The drawing under review shows one solid part. Ordinate dimensions are in mm from its lowest x, y, z. A direction names the side the tool comes from. Give positions to 0.01 mm unless a question says otherwise; leave off trailing zeros. Order: outer loops, then holes, each group sorted by start corner. A loop starts at its lowest first (then second) coordinate and runs counter-clockwise, first axis right, second up. Notation, with made-up numbers: (14, -12) - (58, -12) arc R23 cw to (58, 6) - close; hole circle Ø11 at (7, -12). An arc over 180 degrees is marked (long way). Use CSV: the item, a comma, the result in double quotes. Start each with the question number.
1. Take a section at B-B, the plane z = 105. State the section outline as (x, y) points (1 decimal).
2. Draft analysis for pull direction Z (two halves, no side actions). For the marked faces 1, 2, 3 and 4, state which applies: released by +Z, released by -Z, zero draft, split by the parting line, or undercut.
3. To check wall thickness, follow line 1 (X direction, y = 101, z = 130); line 2 (Y direction, x = 163.5, z = 130); line 3 (Z direction, x = 134, y = 170). State the ranges of each line that lie inside material, in increasing order. Write a range as [from, to].
4. For pin 1 (5 mm diameter, centred on y = 192.5, z = 167.5, fed in from +X); pin 2 (10 mm diameter, centred on x = 213.5, z = 207, fed in from +Y); pin 3 (3 mm diameter, centred on y = 156, z = 71, fed in from -X), all flat-tipped, find the tip position at first contact; note any pin that passes through.
5. Take a section at D-D, the plane z = 150. State the section outline as (x, y) points, then the cut area to 3 significant figures.
6. Take a section at C-C, the plane x = 65. State the section outline as (y, z) points, then the cut area to 3 significant figures.
7. Take a section at A-A, the plane y = 80.5. State the section outline as (x, z) points, then the cut area to 3 significant figures.
8. Machinability: for the marked faces 5, 6 and 7, which of the approach directions +Z, -Z, +X, -X, +Y, -Y give a long, thin tool a straight path to every point of the face, cutting with its end or side? Answer none if there is none.
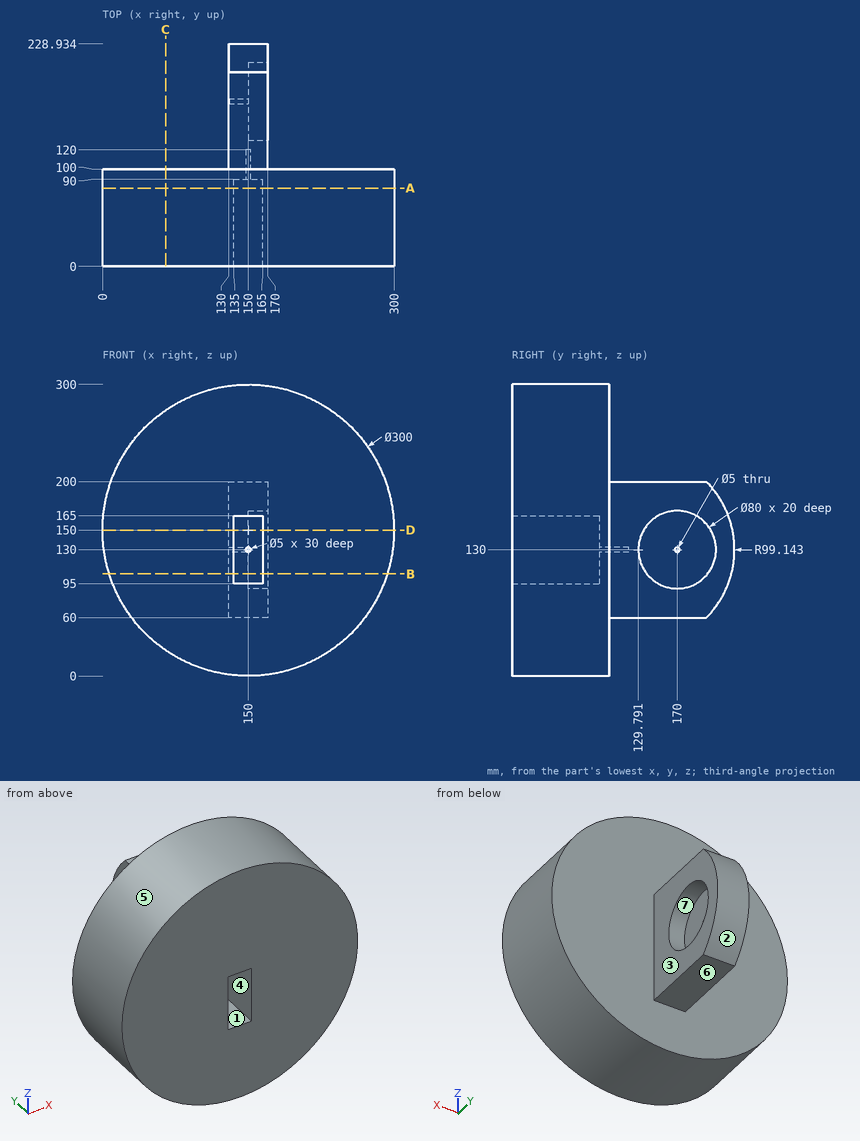
Determined:
1,outline,"(6.9, 0) - (135, 0) - (135, 90) - (165, 90) - (165, 0) - (293.1, 0) - (293.1, 100) - (170, 100) - (170, 138.8) - (150, 138.8) - (150, 201.2) - (170, 201.2) - (170, 225.7) - (130, 225.7) - (130, 100) - (6.9, 100) - close"
2,face 1,"undercut"
2,face 2,"split by the parting line"
2,face 3,"zero draft"
2,face 4,"undercut"
3,line 1,"x = [130, 147.5], [152.5, 170]"
3,line 2,"y = [90, 130], [210, 228.93]"
3,line 3,"z = [60, 127.5], [132.5, 200]"
4,pin 1,"stops at x = 170"
4,pin 2,"stops at y = 100"
4,pin 3,"stops at x = 130"
5,outline,"(0, 0) - (135, 0) - (135, 90) - (165, 90) - (165, 0) - (300, 0) - (300, 100) - (170, 100) - (170, 135.36) - (150, 135.36) - (150, 204.64) - (170, 204.64) - (170, 226.9) - (130, 226.9) - (130, 100) - (0, 100) - close"
5,area,"31,000 mm²"
6,outline,"(0, 26.41) - (100, 26.41) - (100, 273.59) - (0, 273.59) - close"
6,area,"24,700 mm²"
7,outline,"circle Ø300 at (150, 150); hole (135, 95) - (165, 95) - (165, 165) - (135, 165) - close"
7,area,"68,600 mm²"
8,face 5,"+Y, -Y"
8,face 6,"-Z, +X, -X, +Y"
8,face 7,"+X"
